Check sheet for the modelled part. Datum: model origin and axes. Units: mm. Face numbers are marked on the shaded views. A direction names the side the tool comes from. Coordinates: 2 decimals unless noted, no trailing zeros. Loops run counter-clockwise (first coordinate to the right, second up) from the corner with the lowest first, then second, coordinate; pieces in that order, holes last. Notation, with made-up numbers: M 67,6 L 104,6 A16 ccw 104,34 Z; hole C -23,79 d3. An arc over 180 degrees is marked long. Answer as CSV lines item,"result". Start each with the question number.
from build123d import *

# Parameters (mm, degrees)
ESQUISSE2_W        = 10
ESQUISSE2_H        = 10
ESQUISSE2_R        = 2.5
ESQUISSE2_H_2      = 20
BOSS_EXTRU_3_DEPTH = 10


with BuildPart() as part:
    # Esquisse2 → Boss.-Extru.3 (new body)
    # profile 1 of 3: a face of its own
    with BuildSketch(Plane(origin=(0, 0, 0), x_dir=(0, 0, -1), z_dir=(1, 0, 0))):
        Polygon((-22.246371136, 3.5143436), (-37.246371136, 3.5143436), (-37.246371136, -6.4856564), (-22.246371136, -16.4856564), align=None)
    # profile 2 of 3: a face of its own
    with BuildSketch(Plane(origin=(0, 0, 0), x_dir=(0, 0, -1), z_dir=(1, 0, 0))):
        with Locations((-42.246371136, -1.4856564)):
            Rectangle(ESQUISSE2_W, ESQUISSE2_H)
        with Locations((-42.246371136, -1.4856564)):
            Circle(ESQUISSE2_R, mode=Mode.SUBTRACT)
    # profile 3 of 3: a face of its own
    with BuildSketch(Plane(origin=(0, 0, 0), x_dir=(0, 0, -1), z_dir=(1, 0, 0))):
        with Locations((-17.246371136, -6.4856564)):
            Rectangle(ESQUISSE2_W, ESQUISSE2_H_2)
        with Locations((-17.246371136, -11.4856564)):
            Circle(ESQUISSE2_R, mode=Mode.SUBTRACT)
        with Locations((-17.246371136, -1.4856564)):
            Circle(ESQUISSE2_R, mode=Mode.SUBTRACT)
    extrude(amount=BOSS_EXTRU_3_DEPTH)


solid = part.part
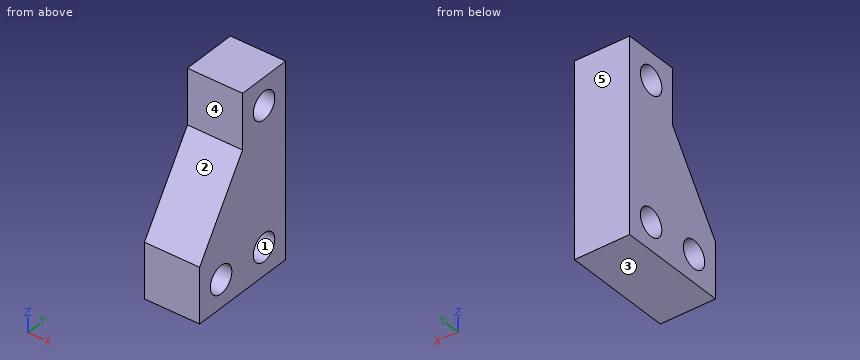
Item 1: Sectioned sample at A-A, the plane z = 16. Record the boundary of the cut face in (x, y), and give its area (3 significant figures).
Item 2: Material ranges on line 1 (Z direction, x = 1.5, y = -1); line 2 (Z direction, x = 1.5, y = 0); line 3 (Y direction, x = 2.25, z = 17.5), recorded low to high. Write a range as from..to.
Item 3: Release check for a two-part mould opening along Y. For the marked faces 1, 2 and 3 record: released by +Y, released by -Y, zero draft, split by the parting line, or undercut.
Item 4: Sectioned sample at D-D, the plane z = 42.5. Record the boundary of the cut face in (x, y), and give its area (3 significant figures).
Item 5: Sectioned sample at B-B, the plane y = -9.5. Record the boundary of the cut face in (x, z).
Item 6: Sectioned sample at C-C, the plane x = 8.75. Record the boundary of the cut face in (y, z).
Item 7: Go/stop test with flat-tipped pins: pin 1 (3 mm diameter, centred on x = 8.5, z = 34, fed in from -Y); pin 2 (3 mm diameter, centred on x = 6.5, z = 39.5, fed in from -Y); pin 3 (4 mm diameter, centred on x = 8.5, y = -13.5, fed in from +Z). Record where each tip stops, or that it passes through.
Item 8: Set-up check for the marked faces 4 and 5: record each of +Z, -Z, +X, -X, +Y, -Y from which the full face is reachable in a straight line by a thin tool's end or side.
Reply:
1,outline,"M 0,-16.49 L 10,-16.49 L 10,-13.65 L 0,-13.65 Z; M 0,-9.32 L 10,-9.32 L 10,-3.65 L 0,-3.65 Z; M 0,0.68 L 10,0.68 L 10,3.51 L 0,3.51 Z"
1,area,"113 mm²"
2,line 1,"12.25..14.79, 19.7..39.79, 44.7..47.25"
2,line 2,"12.25..15.24, 19.26..40.24, 44.26..47.25"
2,line 3,"-16.49..-13.97, -9..-3.97, 1..3.51"
3,face 1,"undercut"
3,face 2,"released by -Y"
3,face 3,"zero draft"
4,outline,"M 0,-6.49 L 10,-6.49 L 10,-3.97 L 0,-3.97 Z; M 0,1 L 10,1 L 10,3.51 L 0,3.51 Z"
4,area,"50.3 mm²"
5,outline,"M 0,12.25 L 10,12.25 L 10,15.73 L 0,15.73 Z; M 0,18.77 L 10,18.77 L 10,32.72 L 0,32.72 Z"
6,outline,"M -16.49,12.25 L 3.51,12.25 L 3.51,47.25 L -6.49,47.25 L -6.49,37.25 L -16.49,22.25 Z; hole C -11.49,17.25 d5; hole C -1.49,17.25 d5; hole C -1.49,42.25 d5"
7,pin 1,"y = -9.65"
7,pin 2,"y = -6.49"
7,pin 3,"z = 29.72"
8,face 4,"+Z, +X, -X, -Y"
8,face 5,"+Z, -Z, +X, -X, +Y"
